```python
from build123d import *

# Parameters (mm, degrees)
SKETCH1_W            = 94
SKETCH1_H            = 66
BOSS_EXTRUDE1_DEPTH  = 2
SKETCH2_W            = 8.8
SKETCH2_H            = 7.9
BOSS_EXTRUDE2_DEPTH  = 8.8
SKETCH3_R            = 2.25
CUT_EXTRUDE1_DEPTH   = 81.055293392
CUT_EXTRUDE2_DEPTH   = 3
CHAMFER1_SIZE        = 1
MIRROR2_COPY_1_DEPTH = 3
CUT_EXTRUDE3_REACH   = 60.099
SKETCH6_W            = 3
SKETCH6_H            = 56


with BuildPart() as part:
    # Sketch1 → Boss-Extrude1 (new body)
    with BuildSketch(Plane(origin=(0, 0, 0), x_dir=(1, 0, 0), z_dir=(0, 1, 0))):
        Rectangle(SKETCH1_W, SKETCH1_H)
    extrude(amount=BOSS_EXTRUDE1_DEPTH)

    # Sketch2 → Boss-Extrude2 (add)
    with BuildSketch(Plane(origin=(0, 2, 0), x_dir=(1, 0, 0), z_dir=(0, 1, 0))):
        with Locations((-40.5, -26.95)):
            Rectangle(SKETCH2_W, SKETCH2_H)
        with Locations((40.5, -26.95)):
            Rectangle(SKETCH2_W, SKETCH2_H)
        with Locations((40.5, 26.95)):
            Rectangle(SKETCH2_W, SKETCH2_H)
        with Locations((-40.5, 26.95)):
            Rectangle(SKETCH2_W, SKETCH2_H)
    extrude(amount=BOSS_EXTRUDE2_DEPTH)

    # Sketch3 → Cut-Extrude1 (cut, through all)
    with BuildSketch(Plane.XY.offset(30.9)):
        with Locations((-40.5, 6.5)):
            Circle(SKETCH3_R)
        with Locations((40.5, 6.5)):
            Circle(SKETCH3_R)
    extrude(amount=-CUT_EXTRUDE1_DEPTH, mode=Mode.SUBTRACT)

    # Sketch5 → Cut-Extrude2 (cut)
    with BuildSketch(Plane.XY.offset(-23)):
        Polygon((-40.5, 10.541451884), (-44, 8.520725942), (-44, 4.479274058), (-40.5, 2.458548116), (-37, 4.479274058), (-37, 8.520725942), align=None)
    cut_extrude2 = extrude(amount=-CUT_EXTRUDE2_DEPTH, mode=Mode.SUBTRACT)

    # Chamfer1
    chamfer1_edges = [part.edges().sort_by_distance(p)[0] for p in [
        (-44.9, 10.8, 26.95),
        (-36.1, 10.8, 26.95),
        (44.9, 10.8, 26.95),
        (36.1, 10.8, 26.95),
        (36.1, 10.8, -26.95),
        (44.9, 10.8, -26.95),
        (-44.9, 10.8, -26.95),
        (-36.1, 10.8, -26.95),
    ]]
    chamfer(chamfer1_edges, length=CHAMFER1_SIZE)

    # Mirror1: Cut-Extrude2 across plane
    add(cut_extrude2.mirror(Plane.XY), mode=Mode.SUBTRACT)

    # Mirror2: Cut-Extrude2 across plane
    add(cut_extrude2.mirror(Plane(origin=(0, 0, 0), x_dir=(0, 0, 1), z_dir=(1, 0, 0))), mode=Mode.SUBTRACT)

    # Mirror2 copy 1 sketch → Mirror2 copy 1 (cut)
    with BuildSketch(Plane(origin=(0, 0, 23), x_dir=(-1, 0, 0), z_dir=(0, 0, -1))):
        Polygon((-40.5, 10.541451884), (-44, 8.520725942), (-44, 4.479274058), (-40.5, 2.458548116), (-37, 4.479274058), (-37, 8.520725942), align=None)
    extrude(amount=-MIRROR2_COPY_1_DEPTH, mode=Mode.SUBTRACT)

    # Sketch6 → Cut-Extrude3 (cut, up to next)
    with BuildSketch(Plane(origin=(0, 2, 0), x_dir=(1, 0, 0), z_dir=(0, 1, 0)), mode=Mode.PRIVATE) as cut_extrude3_sk1:
        with Locations((-3, 0)):
            Rectangle(SKETCH6_W, SKETCH6_H)
    cut_extrude3_tool1 = extrude(cut_extrude3_sk1.sketch, amount=-CUT_EXTRUDE3_REACH, mode=Mode.PRIVATE) & part.part
    # Sketch6 → Cut-Extrude3 (cut, up to next)
    with BuildSketch(Plane(origin=(0, 2, 0), x_dir=(1, 0, 0), z_dir=(0, 1, 0)), mode=Mode.PRIVATE) as cut_extrude3_sk2:
        with Locations((-9, 0)):
            Rectangle(SKETCH6_W, SKETCH6_H)
    cut_extrude3_tool2 = extrude(cut_extrude3_sk2.sketch, amount=-CUT_EXTRUDE3_REACH, mode=Mode.PRIVATE) & part.part
    # Sketch6 → Cut-Extrude3 (cut, up to next)
    with BuildSketch(Plane(origin=(0, 2, 0), x_dir=(1, 0, 0), z_dir=(0, 1, 0)), mode=Mode.PRIVATE) as cut_extrude3_sk3:
        with Locations((-15, 0)):
            Rectangle(SKETCH6_W, SKETCH6_H)
    cut_extrude3_tool3 = extrude(cut_extrude3_sk3.sketch, amount=-CUT_EXTRUDE3_REACH, mode=Mode.PRIVATE) & part.part
    # Sketch6 → Cut-Extrude3 (cut, up to next)
    with BuildSketch(Plane(origin=(0, 2, 0), x_dir=(1, 0, 0), z_dir=(0, 1, 0)), mode=Mode.PRIVATE) as cut_extrude3_sk4:
        with Locations((-21, 0)):
            Rectangle(SKETCH6_W, SKETCH6_H)
    cut_extrude3_tool4 = extrude(cut_extrude3_sk4.sketch, amount=-CUT_EXTRUDE3_REACH, mode=Mode.PRIVATE) & part.part
    # Sketch6 → Cut-Extrude3 (cut, up to next)
    with BuildSketch(Plane(origin=(0, 2, 0), x_dir=(1, 0, 0), z_dir=(0, 1, 0)), mode=Mode.PRIVATE) as cut_extrude3_sk5:
        with Locations((-27, 0)):
            Rectangle(SKETCH6_W, SKETCH6_H)
    cut_extrude3_tool5 = extrude(cut_extrude3_sk5.sketch, amount=-CUT_EXTRUDE3_REACH, mode=Mode.PRIVATE) & part.part
    # Sketch6 → Cut-Extrude3 (cut, up to next)
    with BuildSketch(Plane(origin=(0, 2, 0), x_dir=(1, 0, 0), z_dir=(0, 1, 0)), mode=Mode.PRIVATE) as cut_extrude3_sk6:
        with Locations((3, 0)):
            Rectangle(SKETCH6_W, SKETCH6_H)
    cut_extrude3_tool6 = extrude(cut_extrude3_sk6.sketch, amount=-CUT_EXTRUDE3_REACH, mode=Mode.PRIVATE) & part.part
    # Sketch6 → Cut-Extrude3 (cut, up to next)
    with BuildSketch(Plane(origin=(0, 2, 0), x_dir=(1, 0, 0), z_dir=(0, 1, 0)), mode=Mode.PRIVATE) as cut_extrude3_sk7:
        with Locations((9, 0)):
            Rectangle(SKETCH6_W, SKETCH6_H)
    cut_extrude3_tool7 = extrude(cut_extrude3_sk7.sketch, amount=-CUT_EXTRUDE3_REACH, mode=Mode.PRIVATE) & part.part
    # Sketch6 → Cut-Extrude3 (cut, up to next)
    with BuildSketch(Plane(origin=(0, 2, 0), x_dir=(1, 0, 0), z_dir=(0, 1, 0)), mode=Mode.PRIVATE) as cut_extrude3_sk8:
        with Locations((15, 0)):
            Rectangle(SKETCH6_W, SKETCH6_H)
    cut_extrude3_tool8 = extrude(cut_extrude3_sk8.sketch, amount=-CUT_EXTRUDE3_REACH, mode=Mode.PRIVATE) & part.part
    # Sketch6 → Cut-Extrude3 (cut, up to next)
    with BuildSketch(Plane(origin=(0, 2, 0), x_dir=(1, 0, 0), z_dir=(0, 1, 0)), mode=Mode.PRIVATE) as cut_extrude3_sk9:
        with Locations((21, 0)):
            Rectangle(SKETCH6_W, SKETCH6_H)
    cut_extrude3_tool9 = extrude(cut_extrude3_sk9.sketch, amount=-CUT_EXTRUDE3_REACH, mode=Mode.PRIVATE) & part.part
    # Sketch6 → Cut-Extrude3 (cut, up to next)
    with BuildSketch(Plane(origin=(0, 2, 0), x_dir=(1, 0, 0), z_dir=(0, 1, 0)), mode=Mode.PRIVATE) as cut_extrude3_sk10:
        with Locations((27, 0)):
            Rectangle(SKETCH6_W, SKETCH6_H)
    cut_extrude3_tool10 = extrude(cut_extrude3_sk10.sketch, amount=-CUT_EXTRUDE3_REACH, mode=Mode.PRIVATE) & part.part
    add(cut_extrude3_tool1.solids().sort_by_distance((-3, 2, 0))[0], mode=Mode.SUBTRACT)
    add(cut_extrude3_tool2.solids().sort_by_distance((-9, 2, 0))[0], mode=Mode.SUBTRACT)
    add(cut_extrude3_tool3.solids().sort_by_distance((-15, 2, 0))[0], mode=Mode.SUBTRACT)
    add(cut_extrude3_tool4.solids().sort_by_distance((-21, 2, 0))[0], mode=Mode.SUBTRACT)
    add(cut_extrude3_tool5.solids().sort_by_distance((-27, 2, 0))[0], mode=Mode.SUBTRACT)
    add(cut_extrude3_tool6.solids().sort_by_distance((3, 2, 0))[0], mode=Mode.SUBTRACT)
    add(cut_extrude3_tool7.solids().sort_by_distance((9, 2, 0))[0], mode=Mode.SUBTRACT)
    add(cut_extrude3_tool8.solids().sort_by_distance((15, 2, 0))[0], mode=Mode.SUBTRACT)
    add(cut_extrude3_tool9.solids().sort_by_distance((21, 2, 0))[0], mode=Mode.SUBTRACT)
    add(cut_extrude3_tool10.solids().sort_by_distance((27, 2, 0))[0], mode=Mode.SUBTRACT)


solid = part.part
```
Could you check a few things on this model? Use its own coordinates, in mm. A direction names the side the tool comes from. Coordinates: 2 decimals unless noted, no trailing zeros. Order: outer loops, then holes, each group sorted by start corner. A loop starts at its lowest first (then second) coordinate and runs counter-clockwise, first axis right, second up. Notation, with made-up numbers: M -18,22 L 11,22 A13 ccw 11,26 Z; hole C -6,-5 d2. An arc over 180 degrees is marked long. Use one line per item in the form item = value. Start each with the question number.
1. On a 3-axis mill with a long thin cutter (end or side, diameter ignored), from which of +Z, -Z, +X, -X, +Y, -Y can I reach the whole of each face in a straight line? I mean faces 3 (the flat face through (-25.5, 1, 0)), 4 (the flat face through (42.226, 9.545, -24.479)), 5 (the flat face through (-36.1, 6, 27)), 6 (the flat face through (-39, 3, 23)), 7 (the flat face through (-1, 1, 33)). Say none if no direction works.
2. Suppose I cut it at A-A on x = -27. Write out the boundary of the cut face in (y, z), then the cut area to 3 significant figures.
3. We'd pull the mould along X, two halves only. Please class faces 1 (the flat face through (41, 4, -30.9)), 2 (the flat face through (37, 6, 24)): +X half, -X half, draft (parallel to the pull), parting line (faces both ways), or undercut.
4. Suppose I cut it at B-B on z = -19. Count the separate pieces of the cut face and the enclosed holes in it, then the cut area to 3 significant figures.
5. Please list where these lines run through material, in increasing order: line 1 (X direction, y = 8.5, z = -25); line 2 (Y direction, x = -40.5, z = 28.9); line 3 (Y direction, x = -23, z = -7.5).
6. Suppose I cut it at D-D on x = -0.5. Write out the boundary of the cut face in (y, z).
7. For pin 1 (3.5 mm diameter, centred on y = 6, z = 24.5, fed in from -X); pin 2 (4 mm diameter, centred on x = -34, y = 3, fed in from +Z); pin 3 (1.5 mm diameter, centred on y = 7, z = 25, fed in from +X); pin 4 (3.5 mm diameter, centred on x = -39, y = 5, fed in from +Z), each with a flat end and sliding along its axis, tell me the tip position at first contact or that it passes through.
Geometry says:
q1.face_3 = +Y, -Y
q1.face_4 = none
q1.face_5 = +Z, -Z, +Y
q1.face_6 = +X, -X, +Y
q1.face_7 = +Z, +X, -X, +Y, -Y
q2.outline = M 0,-33 L 2,-33 L 2,-28 L 0,-28 Z; M 0,28 L 2,28 L 2,33 L 0,33 Z
q2.area = 20.0 mm^2
q3.face_1 = draft
q3.face_2 = undercut
q4.separate_pieces = 11
q4.enclosed_holes = 0
q4.area = 128 mm^2
q5.line_1 = -44.9 to -44, -37 to -36.1, 36.1 to 37, 44 to 44.9
q5.line_2 = 0 to 4.25, 8.75 to 10.8
q5.line_3 = 0 to 2
q6.outline = M 0,-33 L 2,-33 L 2,33 L 0,33 Z
q7.pin_1 = -44.9
q7.pin_2 = 33
q7.pin_3 = 44.9
q7.pin_4 = 30.9
